Autodesk Inventor part; units mm, degrees
ref_plane "YZ Plane" through (0, 0, 0) normal (1, 0, 0) x (0, 1, 0)
ref_plane "XZ Plane" through (0, 0, 0) normal (0, 1, 0) x (-1, 0, 0)
ref_plane "XY Plane" through (0, 0, 0) normal (0, 0, 1) x (1, 0, 0)
sketch "Sketch1" plane through (0, 0, 0) normal (0, 0, 1) x (1, 0, 0)
  line L0 (0, 0) -> (60, 0)
  line L1 (60, 0) -> (60, 160)
  line L2 (60, 160) -> (0, 160)
  line L3 (0, 160) -> (0, 0)
  dimension "d0" = 60
  dimension "d1" = 160
extrude "Extrusion1" add sketch "Sketch1" along normal blind 6
sketch "Sketch2" plane through (0, 0, 6) normal (0, 0, 1) x (1, 0, 0)
  line L0 (30, 170) -> (30, -10) construction
  line L1 (14.5, 170) -> (14.5, -10) construction
  line L2 (30, 158) -> (30, 118) construction
  line L3 (18.975, 146.975) -> (18.975, 129.025)
  line L4 (41.025, 129.025) -> (41.025, 146.975)
  arc A0 (41.025, 146.975) -> (18.975, 146.975) centre (30, 146.975) ccw
  arc A1 (18.975, 129.025) -> (41.025, 129.025) centre (30, 129.025) ccw
  line L5 (14.5, 158) -> (14.5, 113) construction
  line L6 (12.75, 156.25) -> (12.75, 114.75)
  line L7 (16.25, 114.75) -> (16.25, 156.25)
  arc A2 (16.25, 156.25) -> (12.75, 156.25) centre (14.5, 156.25) ccw
  arc A3 (12.75, 114.75) -> (16.25, 114.75) centre (14.5, 114.75) ccw
  line L8 (45.5, 158) -> (45.5, 113) construction
  line L9 (47.25, 156.25) -> (47.25, 114.75)
  line L10 (43.75, 114.75) -> (43.75, 156.25)
  arc A4 (47.25, 156.25) -> (43.75, 156.25) centre (45.5, 156.25) ccw
  arc A5 (43.75, 114.75) -> (47.25, 114.75) centre (45.5, 114.75) ccw
  point P0 (0, 0)
  point P1 (30, 138)
  point P2 (14.5, 135.5)
  point P3 (45.5, 135.5)
  dimension "d5" = 15.5
  dimension "d6" = 40
  dimension "d7" = 22.05
  dimension "d8" = 45
  dimension "d9" = 3.5
extrude "Extrusion2" cut sketch "Sketch2" against normal through all
sketch "Sketch3" plane through (0, 0, 6) normal (0, 0, 1) x (1, 0, 0)
  line L0 (60, 160) -> (0, 160)
  line L1 (30, 160) -> (30, 60)
  line L2 (10, 160) -> (8.1852, 108.0317)
  line L3 (10, 160) -> (62, 160) construction
  line L4 (8.1852, 108.0317) -> (0, 108.0317)
  line L5 (0, 160) -> (0, 0)
  line L6 (10, 160) -> (0, 160)
  line L7 (0, 160) -> (0, 108.0317)
  line L8 (50, 160) -> (51.8148, 108.0317)
  line L9 (51.8148, 108.0317) -> (60, 108.0317)
  line L10 (50, 160) -> (60, 160)
  line L11 (60, 160) -> (60, 108.0317)
  dimension "d12" = 100
  dimension "d13" = 52
  dimension "d14" = 92
  dimension "d15" = 92
extrude "Extrusion3" cut sketch "Sketch3" against normal through all
fillet "Fillet1" radius 3 4 edges at (51.8148, 108.0317, 3) (50, 160, 3) (10, 160, 3) (8.1852, 108.0317, 3)
sketch "Sketch4" plane through (0, 0, 6) normal (0, 0, 1) x (1, 0, 0)
  line L0 (30, 0) -> (30, 50)
  line L1 (0, 0) -> (60, 0)
  line L2 (0, 0) -> (7, 0)
  line L3 (7, 0) -> (7, 87)
  line L4 (4, 90) -> (0, 90)
  line L5 (0, 90) -> (0, 0)
  arc A0 (7, 87) -> (4, 90) centre (4, 87) ccw
  point P0 (25, 5)
  point P1 (35, 5)
  point P2 (7, 90)
  dimension "d27" = 7
  dimension "d28" = 90
  dimension "d29" = 3
hole "Hole1" at (25, 5, 6) at (35, 5, 6) direction (0, 0, -1) diameter 4 end through all
extrude "Extrusion4" cut sketch "Sketch4" against normal blind 1.2
sketch "Sketch6" plane through (0, 0, 4.8) normal (0, 0, 1) x (1, 0, 0)
  line L0 (7, 0) -> (0, 0)
  line L1 (0, 108.0317) -> (0, 0)
  point P0 (3.5, 10)
  point P1 (3.5, 25)
  point P2 (3.5, 40)
  point P3 (3.5, 55)
  point P4 (3.5, 70)
  dimension "d32" = 10
  dimension "d33" = 3.5
  dimension "d36" = 15
hole "Hole2" at (3.5, 10, 4.8) at (3.5, 25, 4.8) at (3.5, 40, 4.8) at (3.5, 55, 4.8) at (3.5, 70, 4.8) direction (0, 0, -1) diameter 2 end through all
ref_plane "Work Plane1" through (30, 0, 6) normal (1, 0, 0) x (0, 1, 0)
mirror "Mirror1" about plane through (30, 0, 6) normal (1, 0, 0) of "Extrusion4", "Hole2"
ref_plane "Work Plane2" through (30, 0, 6) normal (1, 0, 0) x (0, 1, 0)
properties part number "Z-baseplate" material "Aluminum 6061"
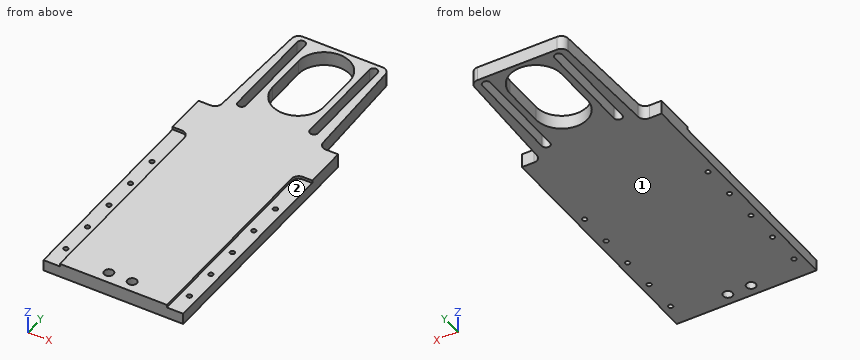
Read the model definition and answer for the solid it produces. Units are mm, in the model's axes. Face numbers are marked on the shaded views. A direction names the side the tool comes from. Coordinates: 2 decimals unless noted, no trailing zeros. Loops run counter-clockwise (first coordinate to the right, second up) from the corner with the lowest first, then second, coordinate; pieces in that order, holes last.
Q1. The part is cut by section A-A on x = 30. Write down the section's boundary in (y, z).
Q2. Consider probe 1 along X at (y, z) = (55, 1.15); probe 2 along Y at (x, z) = (56.5, 3.75); probe 3 along X at (y, z) = (5, 3.5). Determine where each line is inside the solid, lowest interval first.
Q3. Each of these flat-tipped pins is pushed along its axis until it touches: pin 1 Ø1.8 at (x, y) = (3.5, 25) entering from +Z; pin 2 Ø2.5 at (x, y) = (56.5, 70) entering from +Z; pin 3 Ø1.3 at (x, z) = (1.5, 5.5) entering from -Y; pin 4 Ø2.5 at (x, z) = (1.5, 2.5) entering from +Y. Where does it stop, or does it pass through?
Q4. The part is cut by section B-B on y = 44. Write down the section's boundary in (x, z), and give its area (3 significant figures).
Q5. The part is cut by section C-C on y = 122.5. Write down the section's boundary in (x, z).
Q6. The part is cut by section D-D on z = 3.05. Give the number of separate pieces and of enclosed holes in the cut face, and give its area (3 significant figures).
Q7. Which of the six approach directions +Z, -Z, +X, -X, +Y, -Y give full straight-line access (tool end or side, diameter ignored) to the marked faces 1 and 2?
Results below:
1. outline: (0, 0) - (118, 0) - (118, 6) - (0, 6) - close; (158, 0) - (160, 0) - (160, 6) - (158, 6) - close
2. probe 1: x = 0 to 2.5, 4.5 to 55.5, 57.5 to 60
2. probe 2: y = 0 to 9, 11 to 24, 26 to 39, 41 to 54, 56 to 69, 71 to 108.03
2. probe 3: x = 0 to 23, 27 to 33, 37 to 60
3. pin 1: passes through
3. pin 2: stops at z = 4.8
3. pin 3: stops at y = 90
3. pin 4: stops at y = 108.03
4. outline: (0, 0) - (60, 0) - (60, 4.8) - (53, 4.8) - (53, 6) - (7, 6) - (7, 4.8) - (0, 4.8) - close
4. area: 343 mm2
5. outline: (8.69, 0) - (12.75, 0) - (12.75, 6) - (8.69, 6) - close; (16.25, 0) - (21.11, 0) - (21.11, 6) - (16.25, 6) - close; (38.89, 0) - (43.75, 0) - (43.75, 6) - (38.89, 6) - close; (47.25, 0) - (51.31, 0) - (51.31, 6) - (47.25, 6) - close
6. separate pieces: 1
6. enclosed holes: 15
6. area: 7,510 mm2
7. face 1: -Z, +X, -X, +Y, -Y
7. face 2: +Z, +X, -Y
